The listing builds one solid part. Answer for the finished solid, in the listing's coordinates (mm). Round coordinates to 2 decimals unless told otherwise and drop trailing zeros. Order: outer loops, then holes, each group sorted by start corner. A loop starts at its lowest first (then second) coordinate and runs counter-clockwise, first axis right, second up. Notation, with made-up numbers: (5.25, 64) -> (18.25, 64) arc R15 cw to (18.25, 91) -> close; hole circle Ø8 at (81, 47). An arc over 180 degrees is marked (long way). Answer in a Markdown table with one row per item. Add a question column.
```python
from build123d import *

# Parameters (mm, degrees)
SKETCH_1_W      = 7
SKETCH_1_H      = 22
SKETCH_1_R      = 1
SKETCH_1_W_2    = 14
SKETCH_1_R_2    = 1.5
EXTRUDE_1_DEPTH = 3
FILLET_1_R      = 3


with BuildPart() as part:
    # 草图1 → 凸台-拉伸1 (new body)
    # profile 1 of 2: a face of its own
    with BuildSketch(Plane(origin=(0, 0, 0), x_dir=(1, 0, 0), z_dir=(0, 1, 0))):
        Rectangle(SKETCH_1_W, SKETCH_1_H)
        with Locations(Location((0, -7.5, 0), (0, 0, 270))):
            Circle(SKETCH_1_R, mode=Mode.SUBTRACT)
        with Locations(Location((0, 7.5, 0), (0, 0, 270))):
            Circle(SKETCH_1_R, mode=Mode.SUBTRACT)
    # profile 2 of 2: a face of its own
    with BuildSketch(Plane(origin=(0, 0, 0), x_dir=(1, 0, 0), z_dir=(0, 1, 0))):
        with Locations((10.5, 0)):
            Rectangle(SKETCH_1_W_2, SKETCH_1_H)
        with Locations(Location((14, -4, 0), (0, 0, 270))):
            Circle(SKETCH_1_R_2, mode=Mode.SUBTRACT)
        with Locations(Location((14, 4, 0), (0, 0, 270))):
            Circle(SKETCH_1_R_2, mode=Mode.SUBTRACT)
    extrude(amount=EXTRUDE_1_DEPTH)

    # 圆角1
    fillet_1_edges = [part.edges().sort_by_distance(p)[0] for p in [
        (-3.5, 1.5, 11),
        (-3.5, 1.5, -11),
        (17.5, 1.5, -11),
        (17.5, 1.5, 11),
    ]]
    fillet(fillet_1_edges, radius=FILLET_1_R)


solid = part.part
```
Item 1: The part is cut by section B-B, the plane x = 0. Give the vertices of the cut face in (y, z).
Item 2: The part is cut by section D-D, the plane z = -7.5. Give the vertices of the cut face in (x, y).
Item 3: The part is cut by section C-C, the plane y = 1.5. Give the vertices of the cut face in (x, z).
Item 4: The part is cut by section A-A, the plane z = 4. Give the vertices of the cut face in (x, y).
Item 5: A flat-ended cylindrical pin translates along its axis: P1, Ø4, axis at x = 14, z = -4, coming from the -Y side. Find the tip coordinate at first contact, or state that the pin passes through.
Item 6: Find the intervals of material crossed by probe 1 along X at (y, z) = (1.45, 4); probe 2 along X at (y, z) = (1.25, -7.5); probe 3 along Z at (x, y) = (13, 2.6), in increasing order. Write a range as [from, to].
Item 7: For a pull along Z with two mould halves and no side action, classify faces 1 (the face through (16.6, 1.52, 10.14)), 2 (the face through (7, 3, 0)), 3 (the face through (-2.6, 1.52, -10.14)), 4 (the face through (13.425, 1.479, 5.386)) as released by +Z, released by -Z, zero draft, split by the parting line, or undercut.
Resolved:
| question | item | result |
|---|---|---|
| 1 | outline | (0, -11) -> (3, -11) -> (3, -8.5) -> (0, -8.5) -> close; (0, -6.5) -> (3, -6.5) -> (3, 6.5) -> (0, 6.5) -> close; (0, 8.5) -> (3, 8.5) -> (3, 11) -> (0, 11) -> close |
| 2 | outline | (-3.5, 0) -> (-1, 0) -> (-1, 3) -> (-3.5, 3) -> close; (1, 0) -> (17.5, 0) -> (17.5, 3) -> (1, 3) -> close |
| 3 | outline | (-3.5, -8) arc R3 ccw to (-0.5, -11) -> (14.5, -11) arc R3 ccw to (17.5, -8) -> (17.5, 8) arc R3 ccw to (14.5, 11) -> (-0.5, 11) arc R3 ccw to (-3.5, 8) -> close; hole circle Ø2 at (0, -7.5); hole circle Ø2 at (0, 7.5); hole circle Ø3 at (14, -4); hole circle Ø3 at (14, 4) |
| 4 | outline | (-3.5, 0) -> (12.5, 0) -> (12.5, 3) -> (-3.5, 3) -> close; (15.5, 0) -> (17.5, 0) -> (17.5, 3) -> (15.5, 3) -> close |
| 5 | P1 | y = 0 |
| 6 | probe 1 | [-3.5, 12.5], [15.5, 17.5] |
| 6 | probe 2 | [-3.5, -1], [1, 17.5] |
| 6 | probe 3 | [-11, -5.12], [-2.88, 2.88], [5.12, 11] |
| 7 | face 1 | released by +Z |
| 7 | face 2 | zero draft |
| 7 | face 3 | released by -Z |
| 7 | face 4 | undercut |
